Design review of the part built by this model. Coordinates are the model's own, in mm. Face numbers are marked on the shaded views. A direction names the side the tool comes from. Coordinates: 2 decimals unless noted, no trailing zeros. Loops run counter-clockwise (first coordinate to the right, second up) from the corner with the lowest first, then second, coordinate; pieces in that order, holes last. Notation, with made-up numbers: M 88.5,-9 L 135.5,-9 A35 ccw 135.5,25 Z; hole C -35.5,76.25 d11. An arc over 180 degrees is marked long. Put each result on its own line as item: value. Start each with the question number.
(1) Clearance check with flat-ended pins moving along their axes: pin 1 (1.5 mm diameter, centred on x = 192.5, z = 1.5, fed in from +Y); pin 2 (3 mm diameter, centred on y = 195, z = 0, fed in from +X); pin 3 (3 mm diameter, centred on y = 161.5, z = -2, fed in from +X). State where each tip first meets the part, or that it passes through.
(2) Take a section at B-B, the plane x = -195.5. Give the boundary of the cut face in (y, z) (1 decimal).
(3) Take a section at A-A, the plane y = 92. Give the boundary of the cut face in (x, z) (1 decimal).
(4) Take a section at C-C, the plane x = 137.5. Give the boundary of the cut face in (y, z) (3 decimals).
(5) For probe 1 along Y at (x, z) = (-231, 0.5); probe 2 along Z at (x, y) = (-116.5, 29); probe 3 along Y at (x, z) = (66, 0.75), list the stretches that pass through material, from the lowest coordinate up. Write a range as [from, to].
(6) For the marked faces 1, 2 and 3, list the 3-axis set-ups (+Z, -Z, +X, -X, +Y, -Y) from which the entire face can be reached by the end or side of a thin tool; tool diameter is ignored.
(7) Take a section at D-D, the plane y = 189. Give the boundary of the cut face in (x, z) (3 decimals), then the cut area to 3 significant figures.
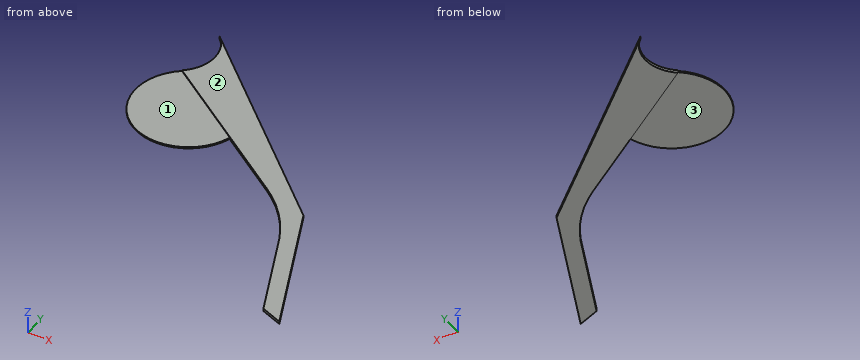
```python
from build123d import *

# Parameters (mm, degrees)
F1_DEPTH      = 1.5875
F1_DEPTH_BACK = 1.5875
F2_DEPTH      = 3.175
F2_DEPTH_BACK = 3.175


with BuildPart() as f1:
    # F0 (on Top) → F1 (new body, two sides)
    with BuildSketch(Plane.XY) as f1_sk:
        with BuildLine():
            ThreePointArc((-240.189908, 141.027898), (-232.480487, -63.960841), (-39.572017, 5.796884))
            Line((-39.572017, 5.796884), (-240.189908, 141.027898))
        make_face()
        with BuildLine():
            ThreePointArc((-39.572017, 5.796884), (-35.770322, 23.39217), (-34.494547, 41.34821))
            ThreePointArc((-34.494547, 41.34821), (-45.59562, 93.275456), (-76.95815, 136.124777))
            ThreePointArc((-76.95815, 136.124777), (-157.681468, 168.290955), (-240.189908, 141.027898))
            Line((-240.189908, 141.027898), (-39.572017, 5.796884))
        make_face()
    extrude(amount=F1_DEPTH)
    extrude(f1_sk.sketch, amount=-F1_DEPTH_BACK)

    # F0 (on Top) → F2 (join, two sides)
    with BuildSketch(Plane.XY) as f2_sk:
        with BuildLine():
            ThreePointArc((-240.189908, 141.027898), (-157.681468, 168.290955), (-76.95815, 136.124777))
            Line((-76.95815, 136.124777), (-236.074097, 278.048981))
            ThreePointArc((-236.074097, 278.048981), (-206.193013, 208.579063), (-240.189908, 141.027898))
        make_face()
        with BuildLine():
            ThreePointArc((-76.95815, 136.124777), (-45.59562, 93.275456), (-34.494547, 41.34821))
            ThreePointArc((-34.494547, 41.34821), (-35.770322, 23.39217), (-39.572017, 5.796884))
            Line((-39.572017, 5.796884), (115.377201, -98.650131))
            ThreePointArc((115.377201, -98.650131), (179.07571, -155.098555), (225.835229, -226.214459))
            Line((225.835229, -226.214459), (321.766937, -439.594988))
            Line((321.766937, -439.594988), (372.139368, -458.721884))
            Line((372.139368, -458.721884), (226.326865, -134.391691))
            Line((226.326865, -134.391691), (-76.95815, 136.124777))
        make_face()
        with BuildLine():
            ThreePointArc((-39.572017, 5.796884), (-35.770322, 23.39217), (-34.494547, 41.34821))
            ThreePointArc((-34.494547, 41.34821), (-45.59562, 93.275456), (-76.95815, 136.124777))
            ThreePointArc((-76.95815, 136.124777), (-157.681468, 168.290955), (-240.189908, 141.027898))
            Line((-240.189908, 141.027898), (-39.572017, 5.796884))
        make_face()
    extrude(amount=F2_DEPTH)
    extrude(f2_sk.sketch, amount=-F2_DEPTH_BACK)


solid = f1.part
```
Computed values:
1. pin 1: stops at y = -103.55
1. pin 2: stops at x = -141.28
1. pin 3: stops at x = -103.73
2. outline: M -81,-1.6 L 110.9,-1.6 L 110.9,-3.2 L 241.9,-3.2 L 241.9,3.2 L 110.9,3.2 L 110.9,1.6 L -81,1.6 Z
3. outline: M -278,-1.6 L -167.5,-1.6 L -167.5,-3.2 L -27.5,-3.2 L -27.5,3.2 L -167.5,3.2 L -167.5,1.6 L -278,1.6 Z
4. outline: M -114.972,-3.175 L -55.162,-3.175 L -55.162,3.175 L -114.972,3.175 Z
5. probe 1: y = [-64.94, 149.38], [273.15, 273.52]
5. probe 2: z = [-1.59, 1.59]
5. probe 3: y = [-65.37, 8.61]
6. face 1: +Z, -X, -Y
6. face 2: +Z, +X, -X, +Y, -Y
6. face 3: -Z, -X, -Y
7. outline: M -208.967,-3.175 L -136.238,-3.175 L -136.238,3.175 L -208.967,3.175 Z
7. area: 462 mm^2
